Study the drawing (mm; zero at the part's minimum x, y, z) and answer. A direction names the side the tool comes from. Coordinates: 2 decimals unless noted, no trailing zeros. Loops run counter-clockwise (first coordinate to the right, second up) from the corner with the lowest first, then second, coordinate; pieces in that order, holes last. Notation, with made-up numbers: (19.25, 6) - (62.25, 6) arc R22 ccw to (62.25, 25) - close; hole circle Ø1 at (31, 59.25). An arc over 180 degrees is marked (long way). Put each result on its own line as item: value.
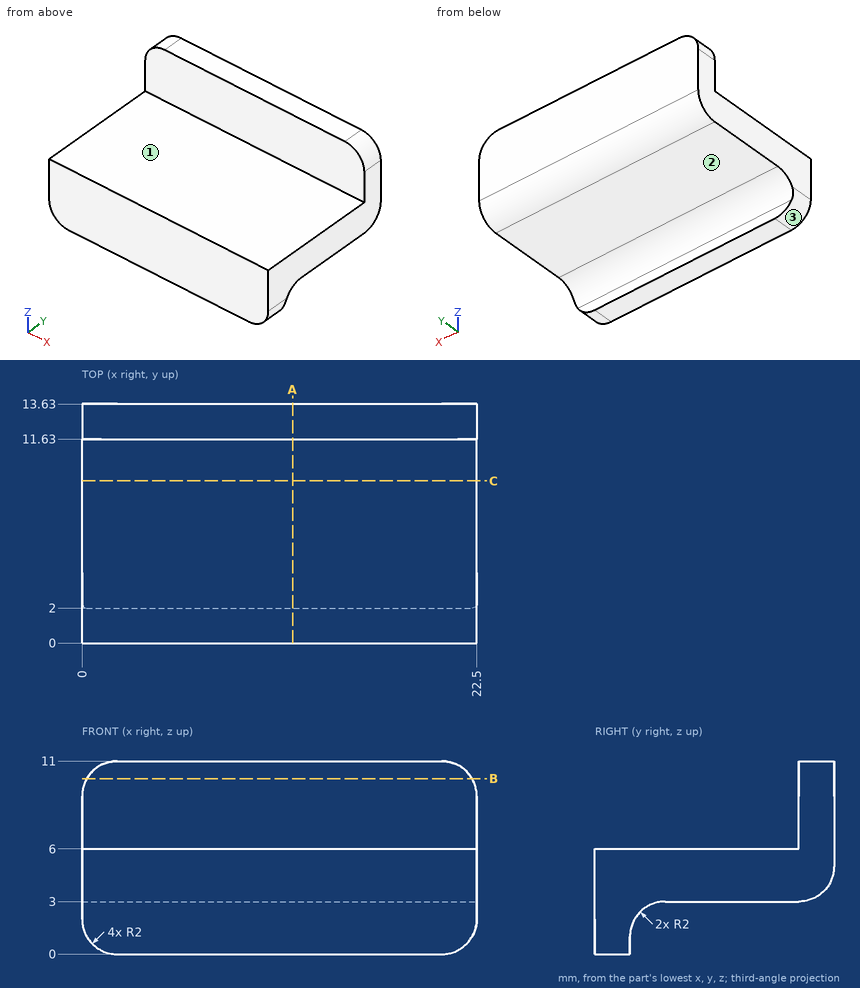
1) The part is cut by section A-A (x = 12). Give the vertices of the cut face in (y, z), and give its area (3 significant figures).
Found:
outline: (0, 0) - (2, 0) - (2, 1) arc R2 cw to (4, 3) - (11.63, 3) arc R2 ccw to (13.63, 5) - (13.63, 11) - (11.63, 11) - (11.63, 6) - (0, 6) - close
area: 56.9 mm^2
2) The part is cut by section C-C (y = 9.25). Give the vertices of the cut face in (x, z).
Found:
outline: (0, 3) - (22.5, 3) - (22.5, 6) - (0, 6) - close
3) For the marked faces 1, 2 and 3, determine the directions among +Z, -Z, +X, -X, +Y, -Y from which every point of the face is accessible in a straight line to the end or side of a thin tool.
Found:
face 1: +Z, +X, -X, -Y
face 2: -Z, +X, -X, +Y
face 3: -Z, -X, +Y, -Y
4) Each of these flat-tipped pins is pushed along its axis until it touches: pin 1 (4 mm diameter, centred on x = 12.5, y = 9.5, fed in from -Z); pin 2 (0.5 mm diameter, centred on x = 6.5, z = 0.5, fed in from +Y); pin 3 (5 mm diameter, centred on x = 11.5, y = 6, fed in from -Z). Where does it stop, or does it pass through?
Found:
pin 1: stops at z = 3
pin 2: stops at y = 2
pin 3: stops at z = 2.94
5) The part is cut by section B-B (z = 10). Give the vertices of the cut face in (x, y), and give its area (3 significant figures).
Found:
outline: (0.27, 11.63) - (22.23, 11.63) - (22.23, 13.63) - (0.27, 13.63) - close
area: 43.9 mm^2
6) Straight lines are drawn through the part: L1, parallel to Y at x = 17.5, z = 9; L2, parallel to Z at x = 3.25, y = 8.5; L3, parallel to Y at x = 10.5, z = 4.5. For each, find the intervals that lie inside material, in ascending order. Write a range as [from, to].
Found:
L1: y = [11.63, 13.63]
L2: z = [3, 6]
L3: y = [0, 13.57]
